Here's the drawing with two shaded views (mm, measured from the low corner). I have some questions. A direction names the side the tool comes from. Give positions to 0.01 mm unless a question says otherwise; leave off trailing zeros. Write each loop counter-clockwise with the first axis right and the second up, starting at its lowest first coordinate (ties: lowest second). Pieces come first, ordered by that corner, then holes. Notation, with made-up numbers: M -32.5,-6 L -22.5,-6 A33 ccw -22.5,31 Z; hole C 3.25,4.25 d5. An arc over 180 degrees is marked long. Use one line per item in the form item = value. Start each with the question number.
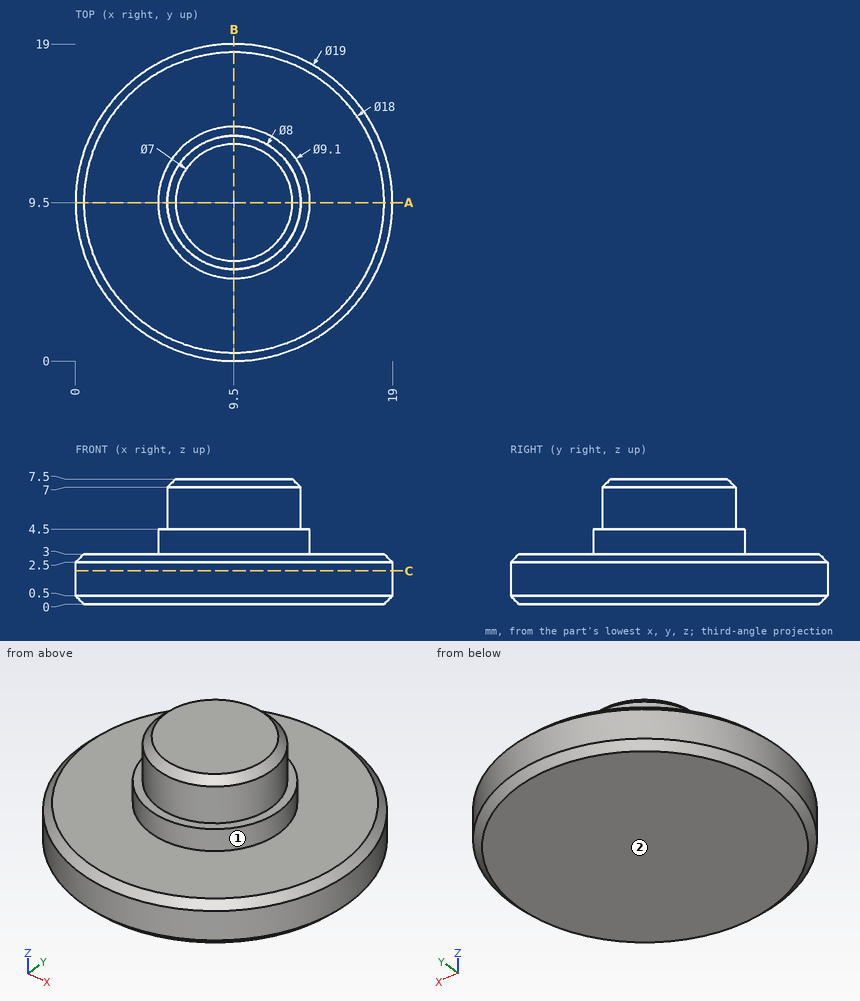
1) Please list where these lines run through material, in increasing order: line 1 (Z direction, x = 17.75, y = 10.5); line 2 (Z direction, x = 7.5, y = 5.5); line 3 (Y direction, x = 9.75, z = 3.75).
2) Suppose I cut it at C-C, the plane z = 2. List the corners of the cut face in (x, y) for me.
3) Suppose I cut it at A-A, the plane y = 9.5. List the corners of the cut face in (x, z) for me, and give its area (3 significant figures).
4) Will these pins go through, and if not, where does the flat tip stop? P1, Ø4, axis at y = 2, z = 4.5, coming from the +X side; P2, Ø2, axis at x = 3, z = 2.5, coming from the +Y side; P3, Ø1.5, axis at x = 14, y = 6, coming from the +Z side.
5) On a 3-axis mill with a long thin cutter (end or side, diameter ignored), from which of +Z, -Z, +X, -X, +Y, -Y can I reach the whole of each face in a straight line? I mean the marked faces 1 and 2. Say none if no direction works.
Checks:
q1.line_1 = 0 to 3
q1.line_2 = 0 to 4.5
q1.line_3 = 4.96 to 14.04
q2.outline = C 9.5,9.5 d19
q3.outline = M 0,0.5 L 0.5,0 L 18.5,0 L 19,0.5 L 19,2.5 L 18.5,3 L 14.05,3 L 14.05,4.5 L 13.5,4.5 L 13.5,7 L 13,7.5 L 6,7.5 L 5.5,7 L 5.5,4.5 L 4.95,4.5 L 4.95,3 L 0.5,3 L 0,2.5 Z
q3.area = 93.9 mm^2
q4.P1 = 16.07
q4.P2 = 17.25
q4.P3 = 3
q5.face_1 = +Z
q5.face_2 = -Z, +X, -X, +Y, -Y
